Check sheet for the modelled part. Datum: model origin and axes. Units: mm. A direction names the side the tool comes from. Coordinates: 2 decimals unless noted, no trailing zeros. Loops run counter-clockwise (first coordinate to the right, second up) from the corner with the lowest first, then second, coordinate; pieces in that order, holes last. Notation, with made-up numbers: M -36.5,34.25 L 4.5,34.25 A15 cw 4.5,47.25 Z; hole C 82,-14 d6. An arc over 180 degrees is marked long. Use CSV: the item, a comma, the result in double quotes. Start each with the question number.
(1) Section check B-B on x = -29.6. Record the cut outline in (y, z).
(2) Section check A-A on z = -3. Record the cut outline in (x, y).
(3) Draft check along Y on faces 1 (the flat face through (-26, -16, 2.5)), 2 (the flat face through (-27, -20, -4)), 3 (the flat face through (-27.5, 7.5, -5)), 4 (the flat face through (-27, 12, -1)). Enter one of: pulls with the +Y half, pulls with the -Y half, needs draft (parallel to the pull), parting line crosses it, or undercut.
(4) Go/stop test with flat-tipped pins: pin 1 Ø0.8 at (x, y) = (-28.5, 7.5) entering from +Z; pin 2 Ø2.5 at (x, y) = (-27, -18) entering from +Z; pin 3 Ø1.5 at (x, z) = (-26.5, -1) entering from +Y; pin 4 Ø1.1 at (x, y) = (-27, 14.5) entering from +Z. Record where each tip stops, or that it passes through.
(5) Set-up check for faces 5 (the flat face through (-27, 15, -3)), 6 (the flat face through (-27.5, 14.5, -5)), 7 (the flat face through (-29, 9, 1.5)): record each of +Z, -Z, +X, -X, +Y, -Y from which the full face is reachable in a straight line by a thin tool's end or side.
(6) Section check D-D on z = -0.25. Record the cut outline in (x, y).
(7) Scan lines: line 1 (Y direction, x = -27.1, z = 1.5); line 2 (Y direction, x = -26.15, z = 1.25); line 3 (Z direction, x = -27.35, y = -2.5). Record each from-to range of solid material in increasing order.
(8) Section check C-C on y = -14. Record the cut outline in (x, z), and give its area (3 significant figures).
from build123d import *

# Parameters (mm, degrees)
BOX155_W               = 13
BOX155_H               = 40
BOX155_DEPTH           = 10
BOX155_PITCH_ANGLE     = -45
BOX163_W               = 12
BOX163_H               = 44
BOX163_DEPTH           = 10
BOX162_W               = 20
BOX162_H               = 44
BOX162_DEPTH           = 10
BOX158_W               = 4
BOX158_H               = 1
BOX158_DEPTH           = 7
BOX160_W               = 4
BOX160_H               = 1
BOX160_DEPTH           = 7
BOX157_W               = 4
BOX157_H               = 2
BOX157_DEPTH           = 7
BOX159_W               = 4
BOX159_H               = 1
BOX159_DEPTH           = 7
BOX156_W               = 4
BOX156_H               = 1
BOX156_DEPTH           = 7
BOX161_W               = 4
BOX161_H               = 7.2
BOX161_DEPTH           = 7
BOX151_W               = 10
BOX151_H               = 2
BOX151_DEPTH           = 7
BOX152_W               = 10
BOX152_H               = 2
BOX152_DEPTH           = 7
BOX153_W               = 10
BOX153_H               = 2
BOX153_DEPTH           = 7
BOX154_W               = 10
BOX154_H               = 2
BOX154_DEPTH           = 7
BOX150_W               = 5
BOX150_H               = 40
BOX150_DEPTH           = 7
CUT064_PITCH_ANGLE     = 90
CUT064_PLACEMENT_ANGLE = -180


with BuildPart() as chamfer_cube001:
    # Box155 → Box155 (new body)
    with BuildSketch(Plane.XY):
        with Locations((6.5, 20)):
            Rectangle(BOX155_W, BOX155_H)
    extrude(amount=BOX155_DEPTH)


with BuildPart() as chamfer_cube001_1:
    # Box155 pitch: moved
    add(chamfer_cube001.part.rotate(Axis((0, 0, 0), (0, 1, 0)), BOX155_PITCH_ANGLE))


with BuildPart() as chamfer_cube001_2:
    # Box155 placement: moved
    add(chamfer_cube001_1.part.moved(Location((-11.69, 0, -1.19))))


with BuildPart() as re_level_edge_clip_block003:
    # Box163 → Box163 (new body)
    with BuildSketch(Plane(origin=(-21.5, -2, -7), x_dir=(1, 0, 0), z_dir=(0, 0, 1))):
        with Locations((6, 22)):
            Rectangle(BOX163_W, BOX163_H)
    extrude(amount=BOX163_DEPTH)


with BuildPart() as re_level_edge_clip_block002:
    # Box162 → Box162 (new body)
    with BuildSketch(Plane(origin=(-19, -2, 3), x_dir=(1, 0, 0), z_dir=(0, 0, 1))):
        with Locations((10, 22)):
            Rectangle(BOX162_W, BOX162_H)
    extrude(amount=BOX162_DEPTH)


with BuildPart() as cube140:
    # Box158 → Box158 (new body)
    with BuildSketch(Plane(origin=(-6, 12, -2), x_dir=(1, 0, 0), z_dir=(0, 0, 1))):
        with Locations((2, 0.5)):
            Rectangle(BOX158_W, BOX158_H)
    extrude(amount=BOX158_DEPTH)


with BuildPart() as cube142:
    # Box160 → Box160 (new body)
    with BuildSketch(Plane(origin=(-6, 36.6, -2), x_dir=(1, 0, 0), z_dir=(0, 0, 1))):
        with Locations((2, 0.5)):
            Rectangle(BOX160_W, BOX160_H)
    extrude(amount=BOX160_DEPTH)


with BuildPart() as cube139:
    # Box157 → Box157 (new body)
    with BuildSketch(Plane(origin=(-6, 8, -2), x_dir=(1, 0, 0), z_dir=(0, 0, 1))):
        with Locations((2, 1)):
            Rectangle(BOX157_W, BOX157_H)
    extrude(amount=BOX157_DEPTH)


with BuildPart() as cube141:
    # Box159 → Box159 (new body)
    with BuildSketch(Plane(origin=(-6, 24.4, -2), x_dir=(1, 0, 0), z_dir=(0, 0, 1))):
        with Locations((2, 0.5)):
            Rectangle(BOX159_W, BOX159_H)
    extrude(amount=BOX159_DEPTH)


with BuildPart() as cube138:
    # Box156 → Box156 (new body)
    with BuildSketch(Plane(origin=(-6, 5, -2), x_dir=(1, 0, 0), z_dir=(0, 0, 1))):
        with Locations((2, 0.5)):
            Rectangle(BOX156_W, BOX156_H)
    extrude(amount=BOX156_DEPTH)


with BuildPart() as extra_holes_for_clips001:
    # Box161 → Box161 (new body)
    with BuildSketch(Plane(origin=(-6, 27.4, -2), x_dir=(1, 0, 0), z_dir=(0, 0, 1))):
        with Locations((2, 3.6)):
            Rectangle(BOX161_W, BOX161_H)
    extrude(amount=BOX161_DEPTH)

    # Fusion056: union Cube140, Cube142, Cube139, Cube141, Cube138
    add(cube140.part)
    add(cube142.part)
    add(cube139.part)
    add(cube141.part)
    add(cube138.part)


with BuildPart() as sphere054:
    # Sphere054 → Sphere054 (revolve)
    with BuildSketch(Plane(origin=(-7.5, 34, 0.5), x_dir=(1, 0, 0), z_dir=(0, -1, 0))):
        with BuildLine():
            ThreePointArc((0, -1.5), (1.5, 0), (0, 1.5))
            Line((0, 1.5), (0, -1.5))
        make_face()
    revolve(axis=Axis((-7.5, 34, 0.5), (0, 0, 1)))


with BuildPart() as holes001:
    # Sphere053 → Sphere053 (revolve)
    with BuildSketch(Plane(origin=(-7.5, 28, 0.5), x_dir=(1, 0, 0), z_dir=(0, -1, 0))):
        with BuildLine():
            ThreePointArc((0, -1.5), (1.5, 0), (0, 1.5))
            Line((0, 1.5), (0, -1.5))
        make_face()
    revolve(axis=Axis((-7.5, 28, 0.5), (0, 0, 1)))

    # Fusion058: union Sphere054
    add(sphere054.part)


with BuildPart() as cube134:
    # Box151 → Box151 (new body)
    with BuildSketch(Plane(origin=(-15, 6, -2), x_dir=(1, 0, 0), z_dir=(0, 0, 1))):
        with Locations((5, 1)):
            Rectangle(BOX151_W, BOX151_H)
    extrude(amount=BOX151_DEPTH)


with BuildPart() as cube135:
    # Box152 → Box152 (new body)
    with BuildSketch(Plane(origin=(-15, 10, -2), x_dir=(1, 0, 0), z_dir=(0, 0, 1))):
        with Locations((5, 1)):
            Rectangle(BOX152_W, BOX152_H)
    extrude(amount=BOX152_DEPTH)


with BuildPart() as cube136:
    # Box153 → Box153 (new body)
    with BuildSketch(Plane(origin=(-15, 25.4, -2), x_dir=(1, 0, 0), z_dir=(0, 0, 1))):
        with Locations((5, 1)):
            Rectangle(BOX153_W, BOX153_H)
    extrude(amount=BOX153_DEPTH)


with BuildPart() as cube137:
    # Box154 → Box154 (new body)
    with BuildSketch(Plane(origin=(-15, 34.6, -2), x_dir=(1, 0, 0), z_dir=(0, 0, 1))):
        with Locations((5, 1)):
            Rectangle(BOX154_W, BOX154_H)
    extrude(amount=BOX154_DEPTH)


with BuildPart() as fusion059:
    # Box150 → Box150 (new body)
    with BuildSketch(Plane(origin=(-5, 0, -2), x_dir=(1, 0, 0), z_dir=(0, 0, 1))):
        with Locations((2.5, 20)):
            Rectangle(BOX150_W, BOX150_H)
    extrude(amount=BOX150_DEPTH)

    # Fusion059: union Cube134, Cube135, Cube136, Cube137
    add(cube134.part)
    add(cube135.part)
    add(cube136.part)
    add(cube137.part)


with BuildPart() as sphere052:
    # Sphere052 → Sphere052 (revolve)
    with BuildSketch(Plane(origin=(-7.5, 11.5, 0.5), x_dir=(1, 0, 0), z_dir=(0, -1, 0))):
        with BuildLine():
            ThreePointArc((0, -1.25), (1.25, 0), (0, 1.25))
            Line((0, 1.25), (0, -1.25))
        make_face()
    revolve(axis=Axis((-7.5, 11.5, 0.5), (0, 0, 1)))


with BuildPart() as copy_edge_clip:
    # Sphere051 → Sphere051 (revolve)
    with BuildSketch(Plane(origin=(-7.5, 6.5, 0.5), x_dir=(1, 0, 0), z_dir=(0, -1, 0))):
        with BuildLine():
            ThreePointArc((0, -1.25), (1.25, 0), (0, 1.25))
            Line((0, 1.25), (0, -1.25))
        make_face()
    revolve(axis=Axis((-7.5, 6.5, 0.5), (0, 0, 1)))

    # Fusion057: union Sphere052
    add(sphere052.part)

    # Fusion060: union Fusion059
    add(fusion059.part)

    # Cut060: cut Holes001
    add(holes001.part, mode=Mode.SUBTRACT)

    # Cut061: cut Extra Holes for Clips001
    add(extra_holes_for_clips001.part, mode=Mode.SUBTRACT)

    # Cut062: cut Re-level Edge Clip Block002
    add(re_level_edge_clip_block002.part, mode=Mode.SUBTRACT)

    # Cut063: cut Re-level Edge Clip Block003
    add(re_level_edge_clip_block003.part, mode=Mode.SUBTRACT)

    # Cut064: cut Chamfer Cube001
    add(chamfer_cube001_2.part, mode=Mode.SUBTRACT)


with BuildPart() as copy_edge_clip_1:
    # Cut064 pitch: moved
    add(copy_edge_clip.part.rotate(Axis((0, 0, 0), (0, 1, 0)), CUT064_PITCH_ANGLE))


with BuildPart() as copy_edge_clip_2:
    # Cut064 placement: moved
    add(copy_edge_clip_1.part.moved(Location((-27, 20, -7))).rotate(Axis((-27, 20, -7), (0, 0, 1)), CUT064_PLACEMENT_ANGLE))


solid = copy_edge_clip_2.part
Outcome:
1,outline,"M -20,-7 L 20,-7 L 20,-2 L 15,-2 L 15,-5 L 14,-5 L 14,0.9 L 12,0.9 L 12,-5 L 10,-5 L 10,0.9 L 8,0.9 L 8,-5 L 7,-5 L 7,-2 L -4.4,-2 L -4.4,-5 L -5.4,-5 L -5.4,0.9 L -7.4,0.9 L -7.4,-5 L -14.6,-5 L -14.6,0.9 L -16.6,0.9 L -16.6,-5 L -17.6,-5 L -17.6,-2 L -20,-2 Z"
2,outline,"M -30,-20 L -25,-20 L -25,-17.6 L -30,-17.6 Z; M -30,-16.6 L -25,-16.6 L -25,-14.6 L -30,-14.6 Z; M -30,-7.4 L -25,-7.4 L -25,-5.4 L -30,-5.4 Z; M -30,-4.4 L -25,-4.4 L -25,7 L -30,7 Z; M -30,8 L -25,8 L -25,10 L -30,10 Z; M -30,12 L -25,12 L -25,14 L -30,14 Z; M -30,15 L -25,15 L -25,20 L -30,20 Z"
3,face 1,"needs draft"
3,face 2,"pulls with the -Y half"
3,face 3,"undercut"
3,face 4,"undercut"
4,pin 1,"stops at z = 1.23"
4,pin 2,"stops at z = -2"
4,pin 3,"stops at y = 14.17"
4,pin 4,"stops at z = 2.5"
5,face 5,"+Z, +X, -X"
5,face 6,"+X, -X"
5,face 7,"+Z, -X, +Y, -Y"
6,outline,"M -30,-16.6 L -25,-16.6 L -25,-14.6 L -26.35,-14.6 A1.3 cw -28.65,-14.6 L -30,-14.6 Z; M -30,-7.4 L -28.65,-7.4 A1.3 cw -26.35,-7.4 L -25,-7.4 L -25,-5.4 L -30,-5.4 Z; M -30,8 L -28.37,8 A1 ccw -26.63,8 L -25,8 L -25,10 L -30,10 Z; M -30,12 L -25,12 L -25,14 L -26.63,14 A1 ccw -28.37,14 L -30,14 Z"
7,line 1,"y = -16.6 to -15.04, -6.96 to -5.4, 7.87 to 10, 12 to 14.13"
7,line 2,"y = -16.6 to -14.6, -7.4 to -5.4, 8 to 10, 12 to 14"
7,line 3,"z = -7 to -2"
8,outline,"M -30,-7 L -25,-7 L -25,-5 L -30,-5 Z"
8,area,"10.0 mm²"
